Verification items for the finished model (mm, model axes). A direction names the side the tool comes from. Round coordinates to 2 decimals unless told otherwise and drop trailing zeros. Loops run counter-clockwise (first coordinate to the right, second up) from the corner with the lowest first, then second, coordinate; pieces in that order, holes last.
from build123d import *

# Parameters (mm, degrees)
F0_R     = 10
F1_DEPTH = 1


with BuildPart() as f1:
    # F0 (on Top) → F1 (new body)
    with BuildSketch(Plane.XY):
        Circle(F0_R)
        Polygon((0, 5.1), (4.850388, 1.575987), (2.997705, -4.125987), (-2.997705, -4.125987), (-4.850388, 1.575987), align=None, mode=Mode.SUBTRACT)
    extrude(amount=F1_DEPTH)


solid = f1.part
1. Scan lines: L1, parallel to X at y = -2.5, z = 0.9; L2, parallel to X at y = 1.75, z = 0.9; L3, parallel to Y at x = 2, z = 0.7. Record each from-to range of solid material in increasing order.
2. Tool access check on faces 5 (the face through (-3.911, -1.315, 0.493)), 6 (the face through (-0.1, -4.3, 0)). Record the directions out of +Z, -Z, +X, -X, +Y, -Y that give a thin tool (end or side, any length) a straight path to the whole face; none if there is none.
3. Section check C-C (z = 0.45). Enter the section's corners in (x, y), then the cut area to 3 significant figures.
4. Section check A-A (y = 0). Enter the section's corners in (x, z).
5. Release check for a two-part mould opening along X. For faces 1 (the face through (-0.1, -4.3, 1)), 2 (the face through (-2.459, 3.313, 0.493)), 3 (the face through (3.937, -1.235, 0.493)), 4 (the face through (-2.17, -9.76, 0.49)) record: released by +X, released by -X, zero draft, split by the parting line, or undercut.
6. Section check D-D (x = 6). Enter the section's corners in (y, z), then the cut area to 3 significant figures.
7. Section check B-B (x = 1.25). Enter the section's corners in (y, z), then the cut area to 3 significant figures.
Taken from the geometry:
1. L1: x = -9.68 to -3.53, 3.53 to 9.68
1. L2: x = -9.85 to -4.61, 4.61 to 9.85
1. L3: y = -9.8 to -4.13, 3.65 to 9.8
2. face 5: +Z, -Z
2. face 6: -Z, +X, -X, +Y, -Y
3. outline: circle Ø20 at (0, 0); hole (-4.85, 1.58) - (-3, -4.13) - (3, -4.13) - (4.85, 1.58) - (0, 5.1) - close
3. area: 252 mm2
4. outline: (-10, 0) - (-4.34, 0) - (-4.34, 1) - (-10, 1) - close; (4.34, 0) - (10, 0) - (10, 1) - (4.34, 1) - close
5. face 1: zero draft
5. face 2: undercut
5. face 3: undercut
5. face 4: split by the parting line
6. outline: (-8, 0) - (8, 0) - (8, 1) - (-8, 1) - close
6. area: 16.0 mm2
7. outline: (-9.92, 0) - (-4.13, 0) - (-4.13, 1) - (-9.92, 1) - close; (4.19, 0) - (9.92, 0) - (9.92, 1) - (4.19, 1) - close
7. area: 11.5 mm2
